The listing builds one solid part. Answer for the finished solid, in the listing's coordinates (mm). Round coordinates to 2 decimals unless told otherwise and drop trailing zeros. Loops run counter-clockwise (first coordinate to the right, second up) from the corner with the lowest first, then second, coordinate; pieces in that order, holes last. Notation, with made-up numbers: (36.5, -17.5) - (68.5, -17.5) arc R14 cw to (68.5, -11.5) - close; hole circle Ø6 at (-21.75, 80). An arc over 180 degrees is marked (long way). Write item = value, one per line. Start each with the question number.
1) Given pin 1 Ø0.6 at (x, z) = (-8, 6) entering from +Y; pin 2 Ø2.5 at (x, z) = (7.5, -6) entering from -Y, each flat-ended and moving along its own axis, determine where each tip first touches the part or whether it passes through.
2) Straight lines are drawn through the part: line 1 along Z through (x, y) = (2, 0.4); line 2 along X through (y, z) = (0.45, -7.25); line 3 along X through (y, z) = (0.4, -6.5). For each, find the intervals that lie inside material, in ascending order.
3) Section B-B, the plane y = 0.95 is taken. Give the number of separate pieces and of enclosed holes in the cut face, and give its area (3 significant figures).
4) Section A-A, the plane x = -5.08 is taken. Determine the outline of the cut face in (y, z).
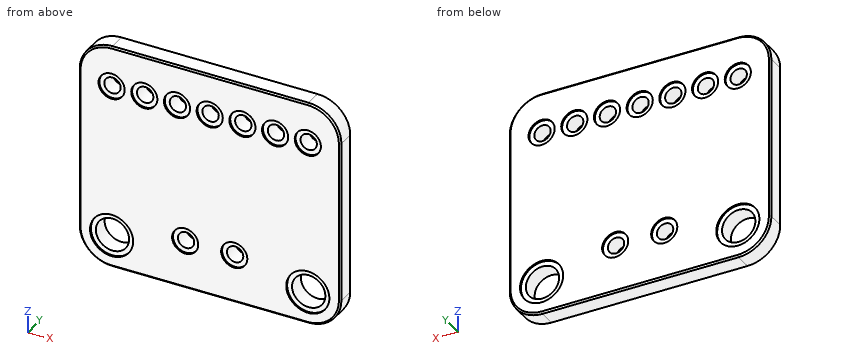
from build123d import *

# Parameters (mm, degrees)
BOSS_EXTRUDE1_DEPTH = 1.524
SKETCH2_R           = 1.294
SKETCH2_R_2         = 0.635
CUT_EXTRUDE1_DEPTH  = 1.524
SKETCH2_4_R         = 1.675
SKETCH2_4_R_2       = 1.016
CUT_EXTRUDE2_DEPTH  = 0.127
CHAMFER1_SIZE       = 0.127


with BuildPart() as part:
    # Sketch1 → Boss-Extrude1 (new body)
    with BuildSketch(Plane(origin=(0, 0, 0), x_dir=(1, 0, 0), z_dir=(0, 1, 0))):
        with BuildLine():
            Line((-7.62, -8.89), (7.62, -8.89))
            ThreePointArc((7.62, -8.89), (9.416051224, -8.146051224), (10.16, -6.35))
            Line((10.16, -6.35), (10.16, 6.35))
            ThreePointArc((10.16, 6.35), (9.416051224, 8.146051224), (7.62, 8.89))
            Line((7.62, 8.89), (-7.62, 8.89))
            ThreePointArc((-7.62, 8.89), (-9.416051224, 8.146051224), (-10.16, 6.35))
            Line((-10.16, 6.35), (-10.16, -6.35))
            ThreePointArc((-10.16, -6.35), (-9.416051224, -8.146051224), (-7.62, -8.89))
        make_face()
    extrude(amount=BOSS_EXTRUDE1_DEPTH)

    # Sketch2 → Cut-Extrude1 (cut)
    with BuildSketch(Plane(origin=(0, 1.524, 0), x_dir=(1, 0, 0), z_dir=(0, 1, 0))):
        with Locations(Location((-7.62, 6.35, 0), (0, 0, 270))):
            Circle(SKETCH2_R)
        with Locations(Location((7.62, 6.35, 0), (0, 0, 270))):
            Circle(SKETCH2_R)
        with Locations(Location((-7.62, -5.715, 0), (0, 0, 270))):
            Circle(SKETCH2_R_2)
        with Locations(Location((-5.08, -5.715, 0), (0, 0, 270))):
            Circle(SKETCH2_R_2)
        with Locations(Location((-2.54, -5.715, 0), (0, 0, 270))):
            Circle(SKETCH2_R_2)
        with Locations(Location((0, -5.715, 0), (0, 0, 270))):
            Circle(SKETCH2_R_2)
        with Locations(Location((2.54, -5.715, 0), (0, 0, 270))):
            Circle(SKETCH2_R_2)
        with Locations(Location((5.08, -5.715, 0), (0, 0, 270))):
            Circle(SKETCH2_R_2)
        with Locations(Location((7.62, -5.715, 0), (0, 0, 270))):
            Circle(SKETCH2_R_2)
        with Locations(Location((1.905, 5.08, 0), (0, 0, 270))):
            Circle(SKETCH2_R_2)
        with Locations(Location((-1.905, 5.08, 0), (0, 0, 270))):
            Circle(SKETCH2_R_2)
    extrude(amount=-CUT_EXTRUDE1_DEPTH, mode=Mode.SUBTRACT)

    # Sketch2_4 → Cut-Extrude2 (cut)
    with BuildSketch(Plane(origin=(0, 1.524, 0), x_dir=(1, 0, 0), z_dir=(0, 1, 0))):
        with Locations(Location((-7.62, 6.35, 0), (0, 0, 270))):
            Circle(SKETCH2_4_R)
        with Locations(Location((7.62, 6.35, 0), (0, 0, 270))):
            Circle(SKETCH2_4_R)
        with Locations(Location((-1.905, 5.08, 0), (0, 0, 270))):
            Circle(SKETCH2_4_R_2)
        with Locations(Location((1.905, 5.08, 0), (0, 0, 270))):
            Circle(SKETCH2_4_R_2)
        with Locations(Location((-7.62, -5.715, 0), (0, 0, 270))):
            Circle(SKETCH2_4_R_2)
        with Locations(Location((-5.08, -5.715, 0), (0, 0, 270))):
            Circle(SKETCH2_4_R_2)
        with Locations(Location((-2.54, -5.715, 0), (0, 0, 270))):
            Circle(SKETCH2_4_R_2)
        with Locations(Location((0, -5.715, 0), (0, 0, 270))):
            Circle(SKETCH2_4_R_2)
        with Locations(Location((2.54, -5.715, 0), (0, 0, 270))):
            Circle(SKETCH2_4_R_2)
        with Locations(Location((5.08, -5.715, 0), (0, 0, 270))):
            Circle(SKETCH2_4_R_2)
        with Locations(Location((7.62, -5.715, 0), (0, 0, 270))):
            Circle(SKETCH2_4_R_2)
    cut_extrude2 = extrude(amount=-CUT_EXTRUDE2_DEPTH, mode=Mode.SUBTRACT)

    # Mirror1: Cut-Extrude2 across plane
    add(cut_extrude2.mirror(Plane.ZX.offset(0.762)), mode=Mode.SUBTRACT)

    # Chamfer1
    chamfer1_edges = [part.edges().sort_by_distance(p)[0] for p in [
        (10.16, 0, 0),
        (9.416051224, 0, 8.146051224),
        (0, 0, 8.89),
        (-9.416051224, 0, 8.146051224),
        (9.416051224, 1.524, 8.146051224),
        (10.16, 1.524, 0),
        (9.416051224, 1.524, -8.146051224),
        (0, 1.524, -8.89),
        (-9.416051224, 1.524, -8.146051224),
        (-10.16, 1.524, 0),
        (-9.416051224, 1.524, 8.146051224),
        (-10.16, 0, 0),
        (0, 1.524, 8.89),
        (-9.416051224, 0, -8.146051224),
        (0, 0, -8.89),
        (9.416051224, 0, -8.146051224),
    ]]
    chamfer(chamfer1_edges, length=CHAMFER1_SIZE)


solid = part.part
Geometry check:
q1.pin_1 = 1.4
q1.pin_2 = 0.13
q2.line_1 = -8.89 to -5.71, -4.45 to 5.38, 6.05 to 8.89
q2.line_2 = -10 to -8.55, -6.69 to 6.69, 8.55 to 10
q2.line_3 = -10.16 to -8.91, -6.33 to 6.33, 8.91 to 10.16
q3.separate_pieces = 1
q3.enclosed_holes = 11
q3.area = 334 mm2
q4.outline = (0, -8.76) - (0.13, -8.89) - (1.4, -8.89) - (1.52, -8.76) - (1.52, 4.7) - (1.4, 4.7) - (1.4, 5.08) - (0.13, 5.08) - (0.13, 4.7) - (0, 4.7) - close; (0, 6.73) - (0.13, 6.73) - (0.13, 6.35) - (1.4, 6.35) - (1.4, 6.73) - (1.52, 6.73) - (1.52, 8.76) - (1.4, 8.89) - (0.13, 8.89) - (0, 8.76) - close
